The model under review builds one solid part; all positions refer to its coordinate system, in mm. Face numbers are marked on the shaded views. A direction names the side the tool comes from. Coordinates: 2 decimals unless noted, no trailing zeros. Loops run counter-clockwise (first coordinate to the right, second up) from the corner with the lowest first, then second, coordinate; pieces in that order, holes last. Notation, with made-up numbers: (-27, -23.5) - (-21, -23.5) arc R6 ccw to (-21, -16.5) - close; hole circle Ø9 at (47, 70.5). An arc over 180 degrees is marked (long way). One line per item, written item: value. Start each with the question number.
1. We need section C-C, the plane y = -14. Give the boundary of the cut face in (x, z).
2. To check wall thickness, follow line 1 (Y direction, x = 25, z = 2.35); line 2 (X direction, y = -21, z = -15); line 3 (Z direction, x = 5.5, y = -61). State the ranges of each line that lie inside material, in increasing order.
3. For the marked faces 1, 2, 3 and 4, list the 3-axis set-ups (+Z, -Z, +X, -X, +Y, -Y) from which the entire face can be reached by the end or side of a thin tool; tool diameter is ignored.
4. Insertion check: P1, Ø13, axis at y = -15.5, z = -13.5, coming from the +X side; P2, Ø12, axis at y = -24.5, z = -7, coming from the +X side; P3, Ø17.5, axis at y = -10.5, z = -20.5, coming from the -X side; P4, Ø8, axis at y = -11.5, z = -20.5, coming from the -X side. Each pin has a flat end and moves straight along its axis. Give the tip position at first contact, or say it passes through.
5. Mouldability with a two-part tool opening along X and no side actions: class the marked faces 5, 6, 7 and 8 as +X half, -X half, draft (parallel to the pull), parting line (faces both ways), or undercut.
6. We need section B-B, the plane z = -22. Count the separate pieces of the cut face and the enclosed holes in it, then the cut area to 3 significant figures.
7. We need section A-A, the plane y = -57. Give the boundary of the cut face in (x, z), then the cut area to 4 significant figures.
8. We need section D-D, the plane z = -5. Give the boundary of the cut face in (x, y).
Autodesk Inventor part; units mm, degrees
ref_plane "Work Plane1" through (30, -28, 0) normal (1, 0, 0) x (0, 0, -1)
ref_plane "YZ Plane" through (0, 0, 0) normal (1, 0, 0) x (0, 1, 0)
ref_plane "XZ Plane" through (0, 0, 0) normal (0, 1, 0) x (-1, 0, 0)
sketch "Sketch1" plane through (0, 0, 0) normal (0, 0, 1) x (1, 0, 0)
  line L0 (-49, 0) -> (49, 0)
  line L1 (-32.5, -75) -> (32.5, -75)
  line L2 (-49, 0) -> (-49, -45)
  line L3 (49, 0) -> (49, -45)
  line L4 (-49, -45) -> (-32.5, -75)
  line L5 (32.5, -75) -> (49, -45)
  point P0 (0, 0)
  point P1 (0, 0)
  point P2 (0, -75)
  dimension "d0" = 98
  dimension "d1" = 65
  dimension "d2" = 75
  dimension "d4" = 45
extrude "Extrusion1" add sketch "Sketch1" along normal blind 5
sketch "Sketch2" plane through (0, 0, 0) normal (0, 0, -1) x (-1, 0, 0)
  line L0 (-25, 0) -> (25, 0) construction
  line L1 (49, 0) -> (-49, 0)
  line L2 (-25, 0) -> (-35, 0)
  line L3 (-35, 0) -> (-35, -28)
  line L4 (-35, -28) -> (-25, -28)
  line L5 (-25, -28) -> (-25, 0)
  point P0 (0, 0)
  point P1 (0, 0)
  dimension "d7" = 50
  dimension "d8" = 10
  dimension "d9" = 28
extrude "Extrusion2" add sketch "Sketch2" along normal blind 25
sketch "Sketch3" plane through (25, -28, 0) normal (-1, 0, 0) x (0, 0, 1)
  line L0 (-25, 0) -> (-25, 28)
  circle A0 centre (-25, 14) radius 11.1125
  point P0 (0, 28)
  dimension "d12" = 22.225
extrude "Extrusion3" cut sketch "Sketch3" against normal through all
ref_plane "Work Plane1" through (30, -28, 0) normal (1, 0, 0) x (0, 0, -1)
sketch "Sketch4" plane through (30, -28, 0) normal (1, 0, 0) x (0, 0, -1)
  arc A0 (25, 25.1125) -> (25, 2.8875) centre (25, 14) ccw
  circle A1 centre (25, 14) radius 14.6312
  point P0 (0, 28)
  point P1 (25, -0.6312)
  point P2 (25, 28.6312)
sketch "Sketch5" plane through (0, 0, -25) normal (0, 0, -1) x (-1, 0, 0)
  line L0 (-28, -27.1312) -> (-32, -27.1312)
  line L1 (-32, -27.1312) -> (-32, -30.1312)
  line L2 (-32, -30.1312) -> (-28, -30.1312)
  line L3 (-28, -30.1312) -> (-28, -27.1312)
  line L4 (-28, -27.1312) -> (-32, -30.1312) construction
  line L5 (-32, -27.1312) -> (-28, -30.1312) construction
  line L6 (68.6, -14) -> (-68.6, -14)
  point P0 (0, 0)
  point P1 (-30, -28.6312)
  dimension "d17" = 4
  dimension "d18" = 3
revolve "Revolution1" cut sketch "Sketch5" angle 360 about axis through (30, -14, -25) along (1, 0, 0)
mirror "Mirror1" about plane through (0, 0, 0) normal (1, 0, 0) of "Extrusion2", "Extrusion3", "Revolution1"
fillet "Fillet1" radius 9.5 4 edges at (-32.5, -75, 2.5) (32.5, -75, 2.5) (49, -45, 2.5) (-49, -45, 2.5)
fillet "Fillet2" radius 3.75 4 edges at (35, -14, 0) (-35, -14, 0) (-30, -28, 0) (30, -28, 0)
thicken "Thicken1" operation add thickness 0.5 both sides no extend neighbours yes toward (0, -0.9485364, 0.316668) faces at (-28.3333, -24.5406, -21.481)
thicken "Thicken2" operation add thickness 0.5 both sides no extend neighbours yes toward (0, -0.8451901, 0.5344658) faces at (28.3333, -23.3922, -19.0607)
sketch "Sketch6" plane through (0, 0, 5) normal (0, 0, 1) x (1, 0, 0)
  arc A0 (-49, -42.5599) -> (-47.8241, -47.1381) centre (-39.5, -42.5599) ccw
  line L0 (-47.8241, -47.1381) -> (-35.207, -70.0782)
  arc A1 (-35.207, -70.0782) -> (-26.8829, -75) centre (-26.8829, -65.5) ccw
  line L1 (-26.8829, -75) -> (26.8829, -75)
  arc A2 (26.8829, -75) -> (35.207, -70.0782) centre (26.8829, -65.5) ccw
  line L2 (35.207, -70.0782) -> (47.8241, -47.1381)
  arc A3 (47.8241, -47.1381) -> (49, -42.5599) centre (39.5, -42.5599) ccw
  line L3 (49, -42.5599) -> (49, 0)
  line L4 (49, 0) -> (-49, 0)
  line L5 (-49, 0) -> (-49, -42.5599)
  point P0 (0, 0)
  point P1 (25, -57)
  point P2 (-33, -59)
  dimension "d26" = 18
  dimension "d27" = 24
  dimension "d28" = 16
  dimension "d29" = 16
hole "Hole1" at (25, -57, 5) direction (0, 0, -1) diameter 13.5 end through all
properties part number "7-8 HandlebarPlate"
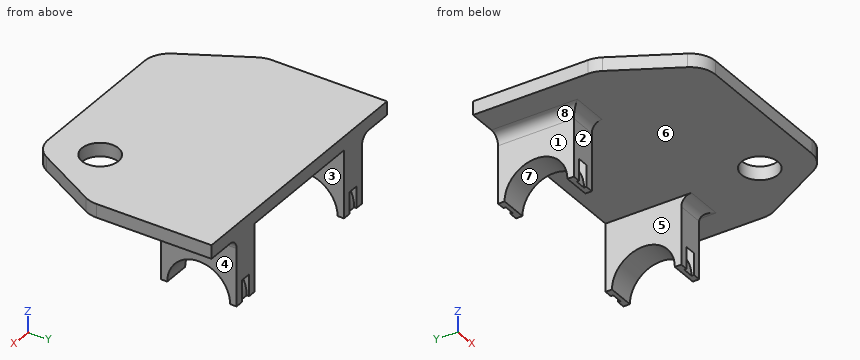
Findings below:
1. outline: (-49, 0) - (-38.75, 0) arc R3.75 cw to (-35, -3.75) - (-35, -13.39) - (-25, -13.39) - (-25, 0) - (25, 0) - (25, -13.39) - (35, -13.39) - (35, -3.75) arc R3.75 cw to (38.75, 0) - (49, 0) - (49, 5) - (-49, 5) - close; hole (-32, -11.87) - (-28, -11.87) - (-28, -8.87) - (-32, -8.87) - close; hole (28, -11.87) - (32, -11.87) - (32, -8.87) - (28, -8.87) - close
2. line 1: -75 to -63.75, -50.25 to 0
2. line 2: -35 to -25, 25 to 35
2. line 3: 0 to 5
3. face 1: -Z, -X, +Y, -Y
3. face 2: -Z, +X, -X, -Y
3. face 3: -Z, +Y, -Y
3. face 4: -Z, +X, +Y, -Y
4. P1: x = 35
4. P2: x = 36.2
4. P3: x = -35
4. P4: through
5. face 5: undercut
5. face 6: undercut
5. face 7: draft
5. face 8: -X half
6. separate pieces: 4
6. enclosed holes: 0
6. area: 91.8 mm2
7. outline: (-42.4, 0) - (18.25, 0) - (18.25, 5) - (-42.4, 5) - close; (31.75, 0) - (42.4, 0) - (42.4, 5) - (31.75, 5) - close
7. area: 356.5 mm2
8. outline: (-35, -28) - (-25, -28) - (-25, 0) - (-35, 0) - close; (25, -28) - (35, -28) - (35, 0) - (25, 0) - close
